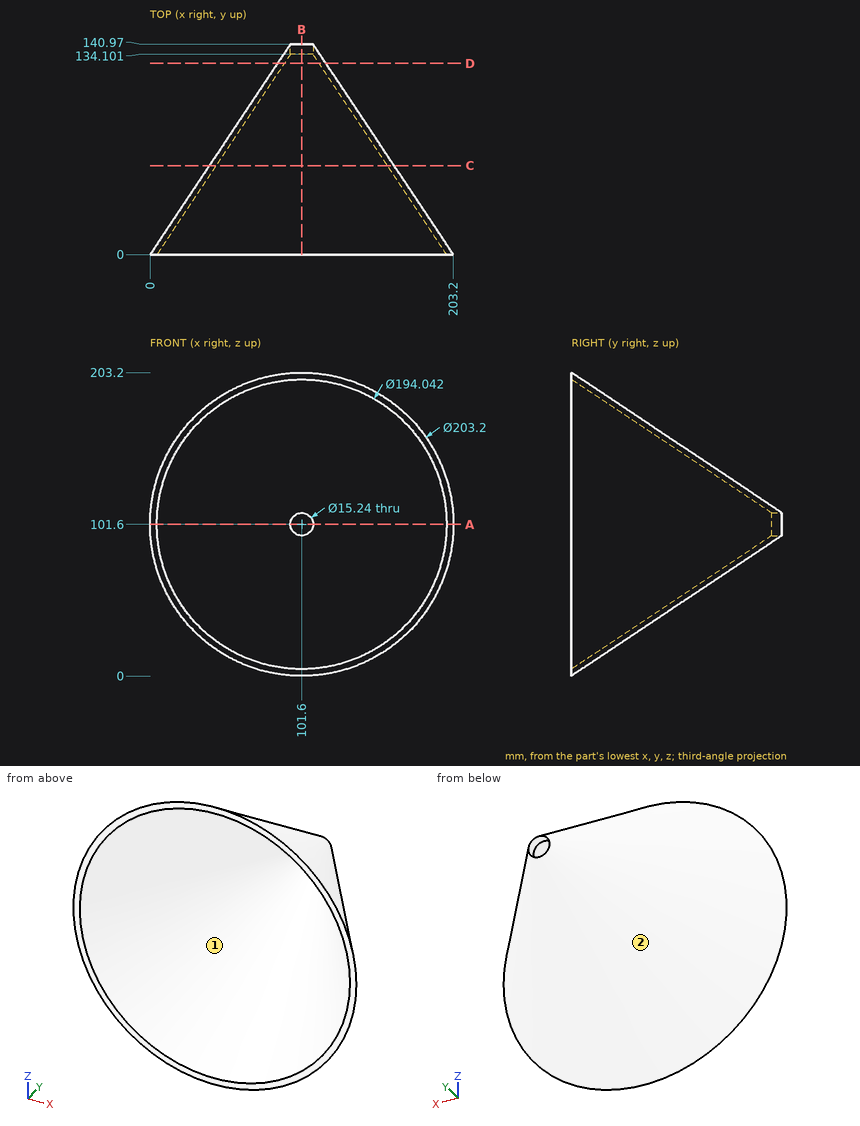
Verification items for this drawing (mm, ordinates from the low corner). Coordinates: 2 decimals unless noted, no trailing zeros. Loops run counter-clockwise (first coordinate to the right, second up) from the corner with the lowest first, then second, coordinate; pieces in that order, holes last.
Item 1: Release check for a two-part mould opening along Z. For the marked faces 1 and 2 record: released by +Z, released by -Z, zero draft, split by the parting line, or undercut.
Item 2: Go/stop test with flat-tipped pins: pin 1 Ø1.5 at (x, z) = (132.5, 77.5) entering from +Y (1 decimal); pin 2 Ø5 at (x, y) = (96, 88.5) entering from -Z; pin 3 Ø1.5 at (x, y) = (82, 51.5) entering from +Z; pin 4 Ø9 at (x, z) = (101.6, 101.6) entering from +Y. Record where each tip stops, or that it passes through.
Item 3: Sectioned sample at C-C, the plane y = 59.5. Record the boundary of the cut face in (x, z) (1 decimal), then the cut area to 3 significant figures.
Item 4: Thickness scan on line 1 (X direction, y = 136, z = 101) (1 decimal); line 2 (X direction, y = 7.5, z = 164.5) (1 decimal); line 3 (Z direction, x = 181, y = 6) (1 decimal). Record the ranges inside material, lowest first.
Item 5: Sectioned sample at D-D, the plane y = 128. Record the boundary of the cut face in (x, z) (1 decimal).
Item 6: Sectioned sample at B-B, the plane x = 101.6. Record the boundary of the cut face in (y, z).
Item 7: Sectioned sample at A-A, the plane z = 101.6. Record the boundary of the cut face in (x, y).
Check result:
1. face 1: undercut
1. face 2: split by the parting line
2. pin 1: stops at y = 94.7
2. pin 2: stops at z = 57.66
2. pin 3: stops at z = 166.52
2. pin 4: passes through
3. outline: circle Ø123.9 at (101.6, 101.6); hole circle Ø114.7 at (101.6, 101.6)
3. area: 1,720 mm2
4. line 1: x = 90.7 to 94, 109.2 to 112.5
4. line 2: x = 28.3 to 34.4, 168.8 to 174.9
4. line 3: z = 44.8 to 53.1, 150.1 to 158.4
5. outline: circle Ø32.5 at (101.6, 101.6); hole circle Ø23.4 at (101.6, 101.6)
6. outline: (0, 0) - (140.97, 93.98) - (134.1, 93.98) - (0, 4.58) - close; (0, 198.62) - (134.1, 109.22) - (140.97, 109.22) - (0, 203.2) - close
7. outline: (0, 0) - (4.58, 0) - (93.98, 134.1) - (93.98, 140.97) - close; (109.22, 134.1) - (198.62, 0) - (203.2, 0) - (109.22, 140.97) - close
